Check sheet for the drawn part. Datum: minimum x, y, z corner. Units: mm. Coordinates: 2 decimals unless noted, no trailing zeros. Loops run counter-clockwise (first coordinate to the right, second up) from the corner with the lowest first, then second, coordinate; pieces in that order, holes last. Notation, with made-up numbers: (42, -12) - (94, -12) arc R22 ccw to (94, 3) - close; hole circle Ø3 at (46.5, 22). An arc over 180 degrees is marked (long way). Answer as CSV lines item,"result". Start each with the question number.
1. Cross-section at D-D (x = 37). Enter the section's corners in (y, z).
2. Cross-section at C-C (z = 7.25). Enter the section's corners in (x, y).
3. Cross-section at A-A (x = 60). Enter the section's corners in (y, z).
4. Material ranges on line 1 (X direction, y = 6.3, z = 6.5); line 2 (Y direction, x = 5, z = 3.25); line 3 (X direction, y = 3.5, z = 6.25), recorded low to high. Write a range as [from, to].
5. Cross-section at B-B (y = 5.5). Enter the section's corners in (x, z), plus the area to 3 significant figures.
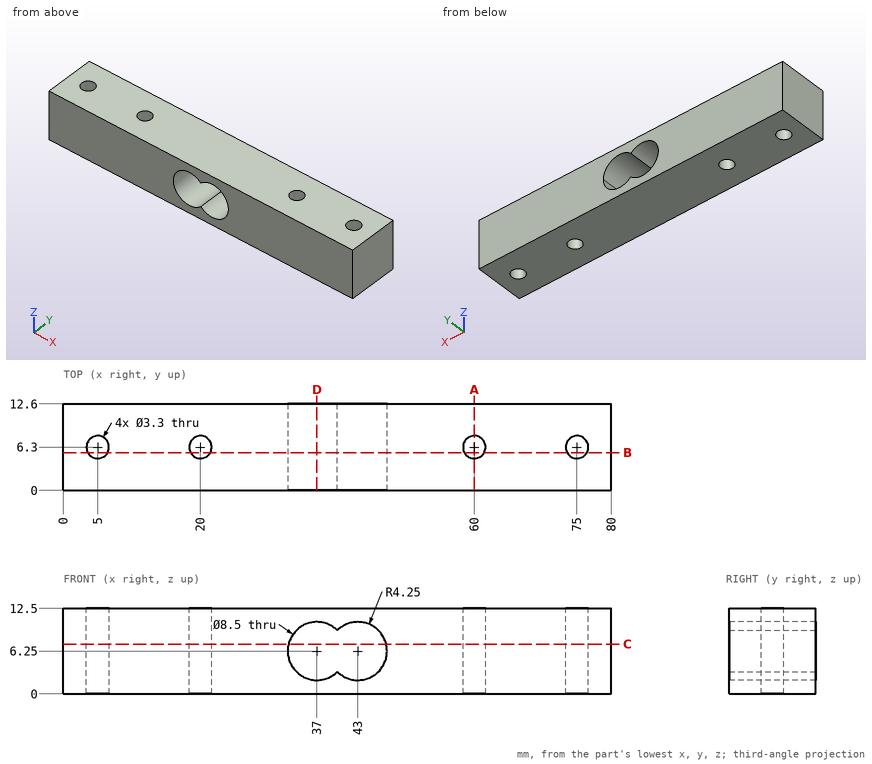
Values follow:
1,outline,"(0, 0) - (12.6, 0) - (12.6, 2) - (0, 2) - close; (0, 10.5) - (12.6, 10.5) - (12.6, 12.5) - (0, 12.5) - close"
2,outline,"(0, 0) - (32.87, 0) - (32.87, 12.6) - (0, 12.6) - close; (47.13, 0) - (80, 0) - (80, 12.6) - (47.13, 12.6) - close; hole circle Ø3.3 at (5, 6.3); hole circle Ø3.3 at (20, 6.3); hole circle Ø3.3 at (60, 6.3); hole circle Ø3.3 at (75, 6.3)"
3,outline,"(0, 0) - (4.65, 0) - (4.65, 12.5) - (0, 12.5) - close; (7.95, 0) - (12.6, 0) - (12.6, 12.5) - (7.95, 12.5) - close"
4,line 1,"x = [0, 3.35], [6.65, 18.35], [21.65, 32.76], [47.24, 58.35], [61.65, 73.35], [76.65, 80]"
4,line 2,"y = [0, 4.65], [7.95, 12.6]"
4,line 3,"x = [0, 32.75], [47.25, 80]"
5,outline,"(0, 0) - (3.56, 0) - (3.56, 12.5) - (0, 12.5) - close; (6.44, 0) - (18.56, 0) - (18.56, 12.5) - (6.44, 12.5) - close; (21.44, 0) - (58.56, 0) - (58.56, 12.5) - (21.44, 12.5) - close; (61.44, 0) - (73.56, 0) - (73.56, 12.5) - (61.44, 12.5) - close; (76.44, 0) - (80, 0) - (80, 12.5) - (76.44, 12.5) - close; hole (40, 3.24) arc R4.25 ccw (long way) to (40, 9.26) arc R4.25 ccw (long way) to start"
5,area,"753 mm²"
